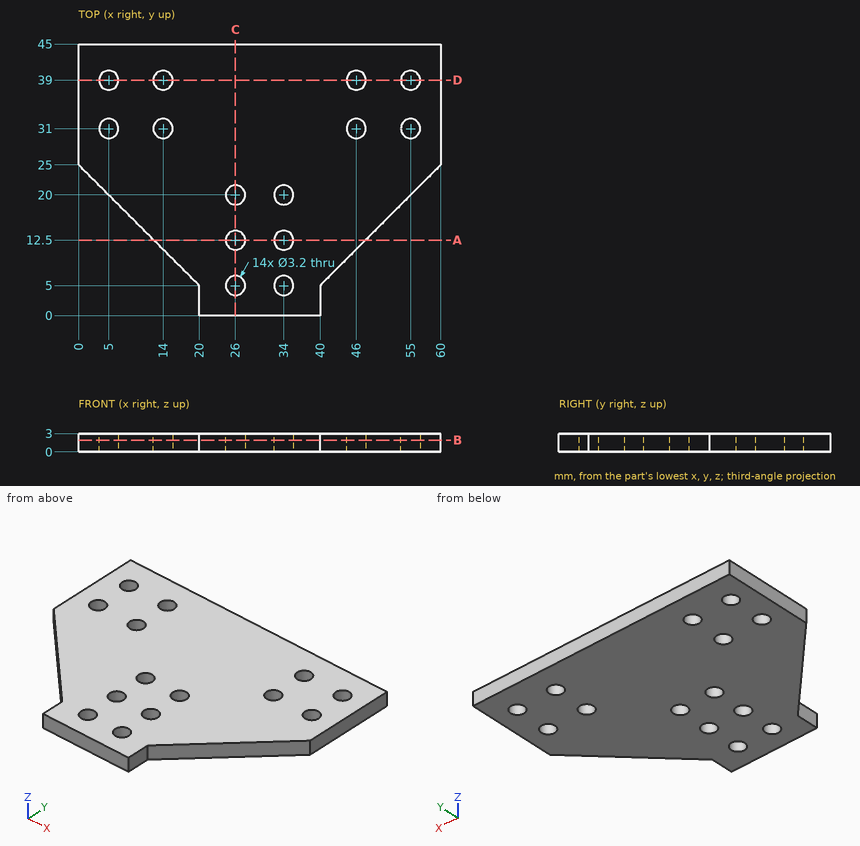
Input: dimensioned drawing with shaded views. Units: mm. Origin: part minimum x, y, z. Give positions to 0.01 mm unless a question says otherwise; leave off trailing zeros. Write each loop counter-clockwise with the first axis right and the second up, starting at its lowest first coordinate (ties: lowest second). Pieces come first, ordered by that corner, then holes.
Q1. First-contact query: P1, Ø0.9, axis at y = 1.5, z = 2, coming from the +X side. Flat tip, straight axial feed; report the tip coordinate or a pass-through.
Q2. Section D-D, the plane y = 39. Output: boundary loops of the cut face in (x, z), plus the area to 3 significant figures.
Q3. Section A-A, the plane y = 12.5. Output: boundary loops of the cut face in (x, z), plus the area to 3 significant figures.
Q4. Material intervals for probe 1 along Y at (x, z) = (26, 0.65); probe 2 along Y at (x, z) = (55, 1.55); probe 3 along X at (y, z) = (30.5, 1.8), sorted ascending.
Q5. Section C-C, the plane x = 26. Output: boundary loops of the cut face in (y, z).
Q6. Section B-B, the plane z = 1.95. State how many separate pieces and enclosed holes the cut face has, plus the area to 3 significant figures.
Filled in:
1. P1: stops at x = 40
2. outline: (0, 0) - (3.4, 0) - (3.4, 3) - (0, 3) - close; (6.6, 0) - (12.4, 0) - (12.4, 3) - (6.6, 3) - close; (15.6, 0) - (44.4, 0) - (44.4, 3) - (15.6, 3) - close; (47.6, 0) - (53.4, 0) - (53.4, 3) - (47.6, 3) - close; (56.6, 0) - (60, 0) - (60, 3) - (56.6, 3) - close
2. area: 142 mm2
3. outline: (12.5, 0) - (24.4, 0) - (24.4, 3) - (12.5, 3) - close; (27.6, 0) - (32.4, 0) - (32.4, 3) - (27.6, 3) - close; (35.6, 0) - (47.5, 0) - (47.5, 3) - (35.6, 3) - close
3. area: 85.8 mm2
4. probe 1: y = 0 to 3.4, 6.6 to 10.9, 14.1 to 18.4, 21.6 to 45
4. probe 2: y = 20 to 29.4, 32.6 to 37.4, 40.6 to 45
4. probe 3: x = 0 to 3.48, 6.52 to 12.48, 15.52 to 44.48, 47.52 to 53.48, 56.52 to 60
5. outline: (0, 0) - (3.4, 0) - (3.4, 3) - (0, 3) - close; (6.6, 0) - (10.9, 0) - (10.9, 3) - (6.6, 3) - close; (14.1, 0) - (18.4, 0) - (18.4, 3) - (14.1, 3) - close; (21.6, 0) - (45, 0) - (45, 3) - (21.6, 3) - close
6. separate pieces: 1
6. enclosed holes: 14
6. area: 1,990 mm2
